CAD build for the part. Positions are in the model's coordinates, mm. A direction names the side the tool comes from. Round coordinates to 2 decimals unless told otherwise and drop trailing zeros. Order: outer loops, then holes, each group sorted by start corner. A loop starts at its lowest first (then second) coordinate and runs counter-clockwise, first axis right, second up. Notation, with made-up numbers: M 11,15 L 57,15 A26 cw 57,29 Z; hole C -32,41.25 d5. An arc over 180 degrees is marked long. Answer as a JSON object with one key per item and string values. Group by question number.
```python
from build123d import *

# Parameters (mm, degrees)
SKETCH1_R           = 4.82599999999999
SKETCH1_R_2         = 4.825999999999997
BOSS_EXTRUDE1_DEPTH = 12.7
SHELL1_T            = -2.0574
FILLET1_R           = 1.27
CUT_EXTRUDE1_DEPTH  = 1714.433575902649
SKETCH3_W           = 21.285199999999943
SKETCH3_H           = 25.40000000000009
CUT_EXTRUDE2_DEPTH  = 1713.0984254933278
FILLET2_R           = 1.27


with BuildPart() as part:
    # Sketch1 → Boss-Extrude1 (new, symmetric)
    with BuildSketch(Plane(origin=(0, -98.29799999999999, -2.776e-14), x_dir=(-1, 0, 0), z_dir=(0, 0, -1))):
        Polygon((32.895539800283125, -12.243824987918671), (1529.236557174524, -143.1567007770127), (1615.5675093984726, -465.34820074258795), (1591.0329934107308, -471.92220448819177), (1509.305208165673, -166.9099575635606), (30.681783934492614, -37.54717031944891), align=None)
        with Locations((41.910000000000004, -25.781000000000002)):
            Circle(SKETCH1_R, mode=Mode.SUBTRACT)
        with Locations((1600.835, -459.4347591199864)):
            Circle(SKETCH1_R_2, mode=Mode.SUBTRACT)
    extrude(amount=BOSS_EXTRUDE1_DEPTH, both=True)

    # Shell1
    shell1_openings = [part.faces().sort_by_distance(p)[0] for p in [
        (-31.788661867, -123.193497654, 0),
        (-1603.300251405, -566.933202615, 0),
        (-1596.009, -557.73275912, 0),
        (-37.084, -124.079, 0),
    ]]
    offset(amount=SHELL1_T, openings=shell1_openings, kind=Kind.INTERSECTION)

    # Fillet1
    fillet1_edges = [part.edges().sort_by_distance(p)[0] for p in [
        (-1572.4020332864984, -402.55045075980036, -12.700000000000028),
        (-1551.9699683205642, -416.485826974324, 10.642599999999971),
        (-1570.6011657541362, -403.77870481135244, 10.642599999999971),
        (-1570.6011657541362, -403.77870481135244, -10.642600000000028),
        (-1551.9699683205642, -416.485826974324, -10.642600000000028),
        (-1572.4020332864984, -402.55045075980036, 12.69999999999997),
        (-1550.1691007882018, -417.71408102587617, 12.69999999999997),
        (-1550.1691007882018, -417.71408102587617, -12.700000000000028),
    ]]
    fillet(fillet1_edges, radius=FILLET1_R)

    # Sketch2 → Cut-Extrude1 (cut, through all)
    with BuildSketch(Plane(origin=(0, 0, -12.700000000000028), x_dir=(-1, 0, 0), z_dir=(0, 0, -1))):
        Polygon((1604.4588423023201, -566.6227591199881), (1590.0690608295056, -566.6227591199881), (1591.0329934107308, -570.2202044881918), align=None)
    extrude(amount=-CUT_EXTRUDE1_DEPTH, mode=Mode.SUBTRACT)

    # Sketch3 → Cut-Extrude2 (cut, through all)
    with BuildSketch(Plane(origin=(0, 0, 0), x_dir=(0, 0, -1), z_dir=(1, 0, 0))):
        with Locations((0, -553.9227591199873)):
            Rectangle(SKETCH3_W, SKETCH3_H)
    extrude(amount=-CUT_EXTRUDE2_DEPTH, mode=Mode.SUBTRACT)

    # Fillet2
    fillet2_edges = [part.edges().sort_by_distance(p)[0] for p in [
        (-1607.836777342822, -541.2227591199872, -10.642599999999971),
        (-1584.9855403231031, -541.2227591199872, -10.642599999999971),
        (-1607.836777342822, -541.2227591199872, 10.642599999999971),
        (-1584.9855403231031, -541.2227591199872, 10.642599999999971),
    ]]
    fillet(fillet2_edges, radius=FILLET2_R - 0.0001)  # a hair under: the kernel refuses the full size


solid = part.part
```
Item 1: Flat gauge pins, fed straight in: pin 1 Ø12 at (y, z) = (-463, -3) entering from +X; pin 2 Ø2.5 at (x, z) = (-1584.5, 2.5) entering from -Y; pin 3 Ø6 at (y, z) = (-389.5, 8) entering from +X; pin 4 Ø12.5 at (x, y) = (-41.91, -124.079) entering from +Z. Where does each tip first touch, or does it go through?
Item 2: Two-plate mould, pull along X, no slides. Class faces 3 (the face through (-1567.803, -394.736, 10.261)), 4 (the face through (-1549.534, -413.869, -12.338)), 5 (the face through (-944, -202, -12.7)), 6 (the face through (-1571.8, -400.3, -0.2)): +X half, -X half, draft (parallel to the pull), parting line (faces both ways), or undercut.
Item 3: 3-axis set-ups, long thin cutter, end or side, ignore diameter. For faces 1 (the face through (-1572.598, -404.679, 12.318)), 2 (the face through (-1566.97, -390.22, -0.13)): which of +Z, -Z, +X, -X, +Y, -Y reach the whole face in a straight line?
Item 4: Cut at B-B, the plane x = -737.5. Give the cut face in (y, z), and give its area (3 significant figures).
Item 5: Cut at A-A, the plane z = -3. Give the cut face in (x, y).
Item 6: Drill centre lines: line 1 (X direction, y = -485, z = -8.5); line 2 (X direction, y = -539.5, z = -6); line 3 (Y direction, x = -208, z = 9.5). Where is each one in solid material? Low to high. Write a range as [from, to].
Response values:
{
 "1": {"pin 1": "x = -1560.7", "pin 2": "y = -541.22", "pin 3": "x = -1541.81", "pin 4": "z = 12.7"},
 "2": {"face 3": "undercut", "face 4": "+X half", "face 5": "draft", "face 6": "-X half"},
 "3": {"face 1": "+Z, -X, +Y", "face 2": "none"},
 "4": {"outline": "M -197.68,-12.7 L -172.19,-12.7 L -172.19,12.7 L -197.68,12.7 Z; hole M -195.62,-10.64 L -174.25,-10.64 L -174.25,10.64 L -195.62,10.64 Z", "area": "193 mm^2"},
 "5": {"outline": "M -1609.56,-541.22 L -1607.43,-541.22 L -1527.62,-243.38 L -32.72,-112.59 L -32.9,-110.54 L -1529.24,-241.45 Z; M -1585.39,-541.22 L -1583.26,-541.22 L -1509.31,-265.21 L -30.68,-135.85 L -30.86,-133.8 L -1510.92,-263.28 Z"},
 "6": {"line 1": "[-1594.49, -1592.36], [-1570.33, -1568.2]", "line 2": "[-1609.1, -1606.97], [-1584.93, -1582.8]", "line 3": "[-151.36, -149.29], [-127.93, -125.86]"}
}
